Could you check a few things on this model? Use its own coordinates, in mm. A direction names the side the tool comes from. Give positions to 0.01 mm unless a question says otherwise; leave off trailing zeros. Loops run counter-clockwise (first coordinate to the right, second up) from the corner with the lowest first, then second, coordinate; pieces in that order, holes last. Notation, with made-up numbers: M 53.5,13.25 L 60.5,13.25 A11 ccw 60.5,21.25 Z; hole C 51.5,74.5 d3. An arc over 180 degrees is marked long. Use CSV: the item, a comma, the result in double quotes.
```python
from build123d import *

# Parameters (mm, degrees)
F1_DEPTH  = 70
F2_DEPTH  = 70
F3_DEPTH  = 40
F4_R      = 25.9673411554
F4_R_2    = 25.5632964649
F5_DEPTH  = 101.6
F5_TAPER  = -7.5
F6_R      = 3.9312257392
F6_R_2    = 4.3669266887
F7_R      = 4.0554960028
F7_R_2    = 4.8000012206
F8_DEPTH  = 25.4
F8_TAPER  = 4
F9_R      = 4.5341790364
F9_R_2    = 4.7105540517
F9_R_3    = 4.7405563192
F9_R_4    = 4.7405580976
F10_DEPTH = 25.4
F10_TAPER = 4


with BuildPart() as f1:
    # F0 (on Right) → F1 (new body)
    with BuildSketch(Plane.YZ):
        with BuildLine():
            Line((0, 56.3131943345), (0, -55.7806827128))
            ThreePointArc((0, -55.7806827128), (17.0028912966, 0.2662558109), (0, 56.3131943345))
        make_face()
    extrude(amount=F1_DEPTH)

    # F2 (add): a face of the model
    f2_faces = [f1.faces().sort_by_distance(p)[0] for p in [
        (0, 6.8528110679, 0.2662558109),
    ]]
    extrude(f2_faces, amount=F2_DEPTH)

    # F3 (add): a face of the model
    f3_faces = [f1.faces().sort_by_distance(p)[0] for p in [
        (0, 0, 0.2662558109),
    ]]
    extrude(f3_faces, amount=F3_DEPTH)

    # F4 (on face) → F5 (cut)
    with BuildSketch(Plane.XZ.offset(40)):
        with Locations((-35.8114647679, 0.6180945247)):
            Circle(F4_R)
        with Locations((36.479592697, 0.1035452609)):
            Circle(F4_R_2)
    extrude(amount=-F5_DEPTH, taper=F5_TAPER, mode=Mode.SUBTRACT)

    # F6 (on face) + F7 (on face) → F8 (cut)
    with BuildSketch(Plane.XZ.offset(40)):
        with Locations((-61.5051910281, 26.2262392789)):
            Circle(F6_R)
        with Locations((-11.1827617511, 26.2262392789)):
            Circle(F6_R_2)
    with BuildSketch(Plane.XZ.offset(40)):
        with Locations((-61.2389370799, -23.5636774451)):
            Circle(F7_R)
        with Locations((-11.1827617511, -23.5636774451)):
            Circle(F7_R_2)
    extrude(amount=-F8_DEPTH, taper=F8_TAPER, mode=Mode.SUBTRACT)

    # F9 (on face) → F10 (cut)
    with BuildSketch(Plane.XZ.offset(40)):
        with Locations((9.8514817655, 26.4924950898)):
            Circle(F9_R)
        with Locations((61.7714524269, 26.4924950898)):
            Circle(F9_R_2)
        with Locations((61.7714524269, -25.6937257946)):
            Circle(F9_R_3)
        with Locations((9.8514817655, -25.6937257946)):
            Circle(F9_R_4)
    extrude(amount=-F10_DEPTH, taper=F10_TAPER, mode=Mode.SUBTRACT)


solid = f1.part
```
1. Please list where these lines run through material, in increasing order: line 1 (X direction, y = -8.5, z = 18); line 2 (X direction, y = -12.5, z = -14); line 3 (Z direction, x = 7, y = -20).
Outcome:
line 1,"-70 to -60.4, -11.22 to 12.76, 60.2 to 70"
line 2,"-70 to -61.54, -10.09 to 10.93, 62.03 to 70"
line 3,"-55.78 to -27.44, -23.95 to 25.19, 27.8 to 56.31"
2. I'm going to push flat-ended pins straight in: pin 1 Ø1.4 at (x, z) = (-62, -24.5) entering from -Y; pin 2 Ø3 at (x, y) = (0.5, 10.5) entering from -Z. Where does each tip first touch, or does it pass through?
Outcome:
pin 1,"y = -14.6"
pin 2,"z = -39.11"
3. I want a section at D-D, the plane y = -10. List the corners of the cut face in (x, z) for me.
Outcome:
outline,"M -70,-55.78 L 70,-55.78 L 70,56.31 L -70,56.31 Z; hole C -35.81,0.62 d59.83; hole C 36.48,0.1 d59.03"
4. I want a section at B-B, the plane y = -26. Give the number of separate pieces and of enclosed holes in the cut face, then the cut area to 3 significant figures.
Outcome:
separate pieces,"1"
enclosed holes,"10"
area,"10,600 mm2"
5. Which directions (+Z, -Z, +X, -X, +Y, -Y) give clear straight access to the entire face, cutting with the end or side of a thin tool? Please do faces 1 (the face through (-11, -14.6, 26)), 2 (the face through (1, -20, 56.313)).
Outcome:
face 1,"-Y"
face 2,"+Z, +X, -X, +Y, -Y"
6. I want a section at A-A, the plane y = 12.5. List the corners of the cut face in (x, z) for me, then the cut area to 3 significant figures.
Outcome:
outline,"M -70,-29.54 L -48.92,-29.54 A32.88 cw -50.43,30.07 L -70,30.07 Z; M -22.71,-29.54 L 23.21,-29.54 A32.48 cw 23.96,30.07 L -21.19,30.07 A32.88 cw Z; M 49,30.07 A32.48 cw 49.75,-29.54 L 70,-29.54 L 70,30.07 Z"
area,"1,840 mm2"
7. If we mould it in two halves opening along Z, with no side actions, what happens to faces 3 (the face through (-1, -20, -55.781)), 4 (the face through (70, -11, 1)), 5 (the face through (-62, -14.6, 26))? For each: +Z half, -Z half, draft (parallel to the pull), parting line (faces both ways), or undercut.
Outcome:
face 3,"-Z half"
face 4,"draft"
face 5,"undercut"
